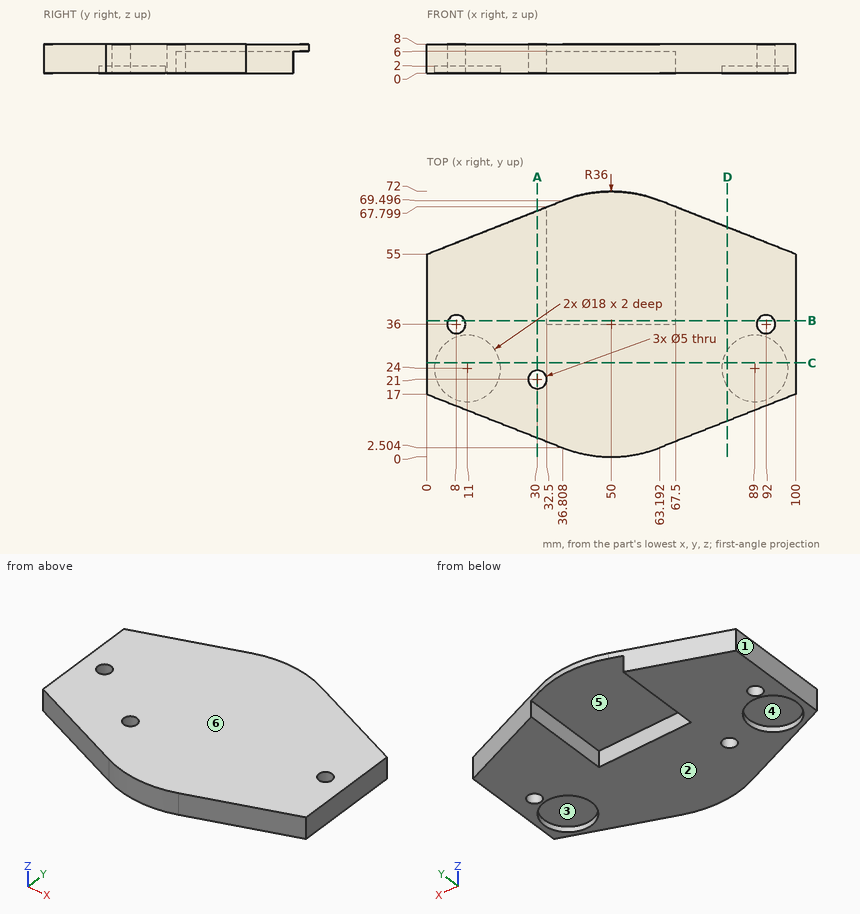
Verification items for this drawing (mm, ordinates from the low corner). A direction names the side the tool comes from. Give positions to 0.01 mm unless a question says otherwise; leave off trailing zeros. Write each loop counter-clockwise with the first axis right and the second up, starting at its lowest first coordinate (ties: lowest second). Pieces come first, ordered by that corner, then holes.
1) Access from +Z, -Z, +X, -X, +Y, -Y to the whole of each face (thin tool, end or side, straight path). Record for the marked faces 5 and 6.
2) Section check C-C, the plane y = 25.5. Record the boundary of the cut face in (x, z) (1 decimal).
3) Gauge pin test, flat ends, axial feed: pin 1 (9 mm diameter, centred on x = 91.5, y = 23.5, fed in from -Z); pin 2 (1.8 mm diameter, centred on x = 54, z = 4, fed in from +Y). Record the tip position at first contact, or that the pin passes through.
4) Section check A-A, the plane x = 30. Record the boundary of the cut face in (y, z) (1 decimal).
5) Section check B-B, the plane y = 37. Record the boundary of the cut face in (x, z).
6) Material ranges on L1, parallel to X at y = 37.5, z = 1.25; L2, parallel to X at y = 51.5, z = 2.5; L3, parallel to Z at x = 58.5, y = 56, recorded low to high.
7) Section check D-D, the plane x = 81.5. Record the boundary of the cut face in (y, z) (1 decimal), and give its area (3 significant figures).
8) Release check for a two-part mould opening along X. For the marked faces 1, 2, 3 and 4 record: pulls with the +X half, pulls with the -X half, needs draft (parallel to the pull), parting line crosses it, or undercut.
Computed:
1. face 5: -Z, +Y
1. face 6: +Z, +X, -X, +Y, -Y
2. outline: (0, 0) - (2.1, 0) - (2.1, 2) - (19.9, 2) - (19.9, 0) - (80.1, 0) - (80.1, 2) - (97.9, 2) - (97.9, 0) - (100, 0) - (100, 8) - (0, 8) - close
3. pin 1: stops at z = 2
3. pin 2: stops at y = 36
4. outline: (5.2, 0) - (18.5, 0) - (18.5, 8) - (5.2, 8) - close; (23.5, 0) - (66.8, 0) - (66.8, 8) - (23.5, 8) - close
5. outline: (0, 0) - (5.71, 0) - (5.71, 8) - (0, 8) - close; (10.29, 0) - (32.5, 0) - (32.5, 6) - (67.5, 6) - (67.5, 0) - (89.71, 0) - (89.71, 8) - (10.29, 8) - close; (94.29, 0) - (100, 0) - (100, 8) - (94.29, 8) - close
6. L1: x = 0 to 6, 10 to 32.5, 67.5 to 90, 94 to 100
6. L2: x = 0 to 32.5, 67.5 to 100
6. L3: z = 6 to 8
7. outline: (9.7, 0) - (19, 0) - (19, 2) - (29, 2) - (29, 0) - (62.3, 0) - (62.3, 8) - (9.7, 8) - close
7. area: 401 mm2
8. face 1: pulls with the -X half
8. face 2: needs draft
8. face 3: undercut
8. face 4: undercut
